Design review of the part built by this model. Coordinates are the model's own, in mm. A direction names the side the tool comes from. Round coordinates to 2 decimals unless told otherwise and drop trailing zeros. Write each loop counter-clockwise with the first axis right and the second up, starting at its lowest first coordinate (ties: lowest second). Pieces come first, ordered by that corner, then holes. Notation, with made-up numbers: (-21.75, 84.25) -> (-3.75, 84.25) arc R21 cw to (-3.75, 90.25) -> close; hole circle Ø8 at (61.5, -39). An arc over 180 degrees is marked (long way). One line per question, with ' | ' between items. Start each with the question number.
1) Consider section A-A (z = 2.75). Give the boundary of the cut face in (x, y) (3 decimals).
2) Consider section D-D (y = 43). Give the boundary of the cut face in (x, z) (3 decimals).
3) Insertion check: pin 1 Ø2 at (x, z) = (119, 1) entering from -Y; pin 2 Ø1.9 at (x, z) = (12.5, 3.5) entering from -Y. Each pin has a flat end and moves straight along its axis. Give the tip position at first contact, or say it passes through.
4) For probe 1 along Y at (x, z) = (112.5, 5.5); probe 2 along Y at (x, z) = (31.5, 5.75); probe 3 along X at (y, z) = (113, 5), list the stretches that pass through material, from the lowest coordinate up.
5) Consider section C-C (x = 95.25). Give the boundary of the cut face in (y, z).
6) Consider section B-B (y = 120.65). Give the boundary of the cut face in (x, z) (3 decimals), then the cut area to 3 significant figures.
7) Mouldability with a two-part tool opening along X and no side actions: class faces 1 (the cylindrical face through (81.209, 133.525, 3.219)), 2 (the flat face through (14, 146.05, 3)), 3 (the flat face through (146.05, 141, 3)) as +X half, -X half, draft (parallel to the pull), parting line (faces both ways), or undercut.
8) For faces 4 (the flat face through (14, 95.25, 3)), 5 (the flat face through (0, 47, 3)), list the 3-axis set-ups (+Z, -Z, +X, -X, +Y, -Y) from which the entire face can be reached by the end or side of a thin tool; tool diameter is ignored.
```python
from build123d import *

# Parameters (mm, degrees)
BOSS_EXTRUDE1_DEPTH = 6.35
SKETCH2_R           = 19.05
CUT_EXTRUDE1_DEPTH  = 7.35


with BuildPart() as part:
    # Sketch1 → Boss-Extrude1 (new body)
    with BuildSketch(Plane.XY):
        Polygon((0, 0), (0, 228.6), (146.05, 228.6), (146.05, 50.8), align=None)
    extrude(amount=BOSS_EXTRUDE1_DEPTH)

    # Sketch2 → Cut-Extrude1 (cut, through all)
    with BuildSketch(Plane.XY.offset(6.35)):
        with Locations((95.25, 120.65)):
            Circle(SKETCH2_R)
        with BuildLine():
            Line((0, 146.05), (28.575, 146.05))
            ThreePointArc((28.575, 146.05), (53.975, 120.65), (28.575, 95.25))
            Line((28.575, 95.25), (0, 95.25))
            ThreePointArc((0, 95.25), (-25.4, 120.65), (0, 146.05))
        make_face()
    extrude(amount=-CUT_EXTRUDE1_DEPTH, mode=Mode.SUBTRACT)


solid = part.part
```
From the geometry:
1) outline: (0, 0) -> (146.05, 50.8) -> (146.05, 228.6) -> (0, 228.6) -> (0, 146.05) -> (28.575, 146.05) arc R25.4 cw to (28.575, 95.25) -> (0, 95.25) -> close; hole circle Ø38.1 at (95.25, 120.65)
2) outline: (0, 0) -> (123.625, 0) -> (123.625, 6.35) -> (0, 6.35) -> close
3) pin 1: stops at y = 41.04 | pin 2: stops at y = 4.02
4) probe 1: y = 39.13 to 112.57, 128.73 to 228.6 | probe 2: y = 10.96 to 95.42, 145.88 to 228.6 | probe 3: x = 52.8 to 77.8, 112.7 to 146.05
5) outline: (33.13, 0) -> (101.6, 0) -> (101.6, 6.35) -> (33.13, 6.35) -> close; (139.7, 0) -> (228.6, 0) -> (228.6, 6.35) -> (139.7, 6.35) -> close
6) outline: (53.975, 0) -> (76.2, 0) -> (76.2, 6.35) -> (53.975, 6.35) -> close; (114.3, 0) -> (146.05, 0) -> (146.05, 6.35) -> (114.3, 6.35) -> close | area: 343 mm2
7) face 1: undercut | face 2: draft | face 3: +X half
8) face 4: +Z, -Z, -X | face 5: +Z, -Z, -X, +Y, -Y
